Could you check a few things on this model? Use its own coordinates, in mm. A direction names the side the tool comes from. Give positions to 0.01 mm unless a question says otherwise; leave off trailing zeros. Loops run counter-clockwise (first coordinate to the right, second up) from the corner with the lowest first, then second, coordinate; pieces in that order, holes last. Notation, with made-up numbers: (-31, -20) - (0, -20) arc R12 cw to (0, -16) - close; hole circle Ø10 at (-3.75, -38). An arc over 180 degrees is marked (long way). Write each question's results on one line, items separated by ' | '. Start each with the question number.
1) I'm going to push flat-ended pins straight in: pin 1 (0.9 mm diameter, centred on x = -7, y = 3.5, fed in from +Z); pin 2 (3 mm diameter, centred on x = -6, z = 3, fed in from +Y); pin 3 (2 mm diameter, centred on x = 7, y = 3.5, fed in from +Z); pin 4 (2 mm diameter, centred on y = 2, z = 1, fed in from +X). Where does each tip first touch, or does it pass through?
2) If we mould it in two halves opening along X, with no side actions, what happens to faces 3 (the face through (-3, -2, 5)), 4 (the face through (-2.17, -9.76, 0.99)), 5 (the face through (-0.163, -7.732, 0.986))? For each: +X half, -X half, draft (parallel to the pull), parting line (faces both ways), or undercut.
3) If I drill on probe 1 along Y at (x, z) = (0, 1.25); probe 2 along Y at (x, z) = (0, 3); probe 3 along Z at (x, y) = (1.75, -6.5), over which ranges is the centre line in solid material (lowest first)? Write a range as [from, to].
4) I want a section at A-A, the plane y = 0. Count the separate pieces of the cut face and the enclosed holes in it, and give its area (3 significant figures).
5) I want a section at C-C, the plane z = 3.9. Write out the boundary of the cut face in (x, y).
6) On a 3-axis mill with a long thin cutter (end or side, diameter ignored), from which of +Z, -Z, +X, -X, +Y, -Y can I reach the whole of each face in a straight line? I mean faces 1 (the face through (2.75, -6.97, 0.99)), 2 (the face through (1, -1, 2)). Say none if no direction works.
from build123d import *

# Parameters (mm, degrees)
SKETCH_R      = 10
SKETCH_R_2    = 0.75
PAD_DEPTH     = 2
SKETCH001_R   = 4.5
SKETCH001_R_2 = 3
PAD001_DEPTH  = 3
SKETCH003_R   = 1.25
POCKET_DEPTH  = 5
FILLET_R      = 0.2


with BuildPart() as part:
    # Sketch → Pad (new body)
    with BuildSketch(Plane.XY):
        Circle(SKETCH_R)
        with Locations((0, 7)):
            Circle(SKETCH_R_2, mode=Mode.SUBTRACT)
        with Locations((3.5, 7)):
            Circle(SKETCH_R_2, mode=Mode.SUBTRACT)
        with Locations((-3.5, 7)):
            Circle(SKETCH_R_2, mode=Mode.SUBTRACT)
        with Locations((-7, 3.5)):
            Circle(SKETCH_R_2, mode=Mode.SUBTRACT)
        with Locations((-7, 0)):
            Circle(SKETCH_R_2, mode=Mode.SUBTRACT)
        with Locations((-7, -3.5)):
            Circle(SKETCH_R_2, mode=Mode.SUBTRACT)
        with Locations((7, 3.5)):
            Circle(SKETCH_R_2, mode=Mode.SUBTRACT)
        with Locations((7, 0)):
            Circle(SKETCH_R_2, mode=Mode.SUBTRACT)
        with Locations((7, -3.5)):
            Circle(SKETCH_R_2, mode=Mode.SUBTRACT)
        with Locations((0, -7)):
            Circle(SKETCH_R_2, mode=Mode.SUBTRACT)
        with Locations((3.5, -7)):
            Circle(SKETCH_R_2, mode=Mode.SUBTRACT)
        with Locations((-3.5, -7)):
            Circle(SKETCH_R_2, mode=Mode.SUBTRACT)
    extrude(amount=PAD_DEPTH)

    # Sketch001 (on Face15 of Pad) → Pad001 (join)
    with BuildSketch(Plane.XY.offset(2)):
        Circle(SKETCH001_R)
        Circle(SKETCH001_R_2, mode=Mode.SUBTRACT)
    extrude(amount=PAD001_DEPTH)

    # Sketch003 → Pocket (cut)
    with BuildSketch(Plane.XY):
        Circle(SKETCH003_R)
    extrude(amount=POCKET_DEPTH, mode=Mode.SUBTRACT)

    # Fillet
    fillet_edges = [part.edges().sort_by_distance(p)[0] for p in [
        (-10, 0, 0),
        (-10, 0, 2),
        (-4.5, 0, 5),
        (-3, 0, 5),
    ]]
    fillet(fillet_edges, radius=FILLET_R)


solid = part.part
Answers:
1) pin 1: passes through | pin 2: stops at y = 8.64 | pin 3: stops at z = 2 | pin 4: stops at x = 9.95
2) face 3: draft | face 4: parting line | face 5: undercut
3) probe 1: y = [-10, -7.75], [-6.25, -1.25], [1.25, 6.25], [7.75, 10] | probe 2: y = [-4.5, -3], [3, 4.5] | probe 3: z = [0, 2]
4) separate pieces: 4 | enclosed holes: 0 | area: 37.9 mm2
5) outline: circle Ø9 at (0, 0); hole circle Ø6 at (0, 0)
6) face 1: +Z, -Z | face 2: +Z
